The model under review builds one solid part; all positions refer to its coordinate system, in mm. Face numbers are marked on the shaded views. A direction names the side the tool comes from. Round coordinates to 2 decimals unless told otherwise and drop trailing zeros. Write each loop counter-clockwise with the first axis right and the second up, starting at its lowest first coordinate (ties: lowest second). Pieces come first, ordered by that corner, then holes. Notation, with made-up numbers: (54, -31.75) - (70, -31.75) arc R33 cw to (70, 1.25) - close; hole circle Ø2 at (28, 42). An arc over 180 degrees is marked (long way). Return JSON: item names as keys, results as strings.
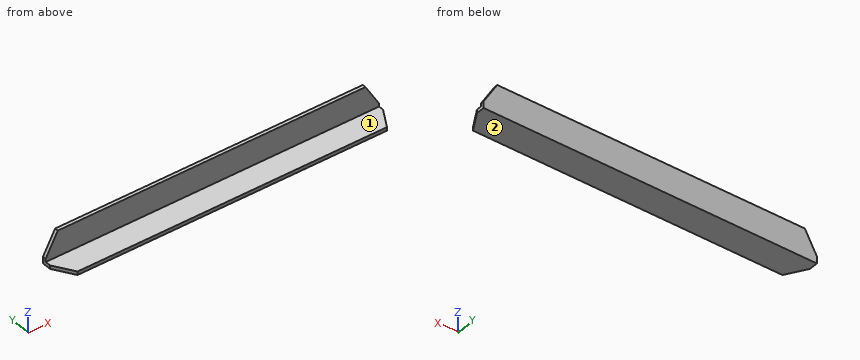
from build123d import *

# Parameters (mm, degrees)
F0_W      = 294.42918
F0_H      = 25.4
F1_DEPTH  = 3.048
F2_W      = 294.42918
F2_H      = 3.048
F3_DEPTH  = 22.352
F5_DEPTH  = 25.4
F7_DEPTH  = 25.4
F9_DEPTH  = 25.4
F11_DEPTH = 25.4


with BuildPart() as f1:
    # F0 (on Front) → F1 (new body)
    with BuildSketch(Plane.XZ):
        with Locations((147.21459, 12.7)):
            Rectangle(F0_W, F0_H)
    extrude(amount=F1_DEPTH)

    # F2 (on face) → F3 (join)
    with BuildSketch(Plane.XZ.offset(3.048)):
        with Locations((147.21459, 1.524)):
            Rectangle(F2_W, F2_H)
    extrude(amount=F3_DEPTH)

    # F4 (on face) → F5 (cut)
    with BuildSketch(Plane.XZ.offset(3.048)):
        Polygon((0, 5.934239), (10.683293, 25.4), (4.401662, 35.47851), (-15.100691, 25.4), align=None)
    extrude(amount=-F5_DEPTH, mode=Mode.SUBTRACT)

    # F6 (on face) → F7 (cut)
    with BuildSketch(Plane.XY.offset(3.048)):
        Polygon((13.454681, -30.058125), (0, -8.04578), (-4.952007, -25.4), (9.960025, -44.26622), align=None)
    extrude(amount=-F7_DEPTH, mode=Mode.SUBTRACT)

    # F8 (on face) → F9 (cut)
    with BuildSketch(Plane.XY.offset(3.048)):
        Polygon((299.843073, 0), (294.42918, -7.468464), (280.858219, -30.611685), (297.753662, -36.44076), align=None)
    extrude(amount=-F9_DEPTH, mode=Mode.SUBTRACT)

    # F10 (on face) → F11 (cut)
    with BuildSketch(Plane.XZ.offset(3.048)):
        Polygon((279.356599, 30.402403), (294.42918, 5.696148), (301.659763, 3.048), (311.673284, 34.467302), align=None)
    extrude(amount=-F11_DEPTH, mode=Mode.SUBTRACT)


solid = f1.part
(1) Add section C-C (z = 14.5). Write out the cut boundary in (x, y), plus the area to 3 significant figures.
Filled in:
{"outline": "(4.7, -3.05) - (289.06, -3.05) - (289.06, 0) - (4.7, 0) - close", "area": "867 mm2"}
(2) For the marked faces 1 and 2, list the 3-axis set-ups (+Z, -Z, +X, -X, +Y, -Y) from which the entire face can be reached by the end or side of a thin tool; tool diameter is ignored.
Filled in:
{"face 1": "+Z, +X, -X, -Y", "face 2": "-Z, +X, -X, +Y, -Y"}
(3) Clearance check with flat-ended pins moving along their axes: pin 1 Ø12 at (x, z) = (218, 22) entering from -Y; pin 2 Ø8 at (y, z) = (-16, 8) entering from +X; pin 3 Ø1 at (x, y) = (33, -17.5) entering from +Z. State where each tip first meets the part, or that it passes through.
Filled in:
{"pin 1": "stops at y = -3.05", "pin 2": "passes through", "pin 3": "stops at z = 3.05"}
(4) Wall thickness on line 1 (Z direction, x = 136, y = -3.25); line 2 (Y direction, x = 204.5, z = 6.75); line 3 (X direction, y = -16.25, z = 2.5): over which ranges is each line inside the solid? List them lowest first.
Filled in:
{"line 1": "z = 0 to 3.05", "line 2": "y = -3.05 to 0", "line 3": "x = 5.01 to 289.28"}
(5) Add section B-B (y = -20). Write out the cut boundary in (x, z).
Filled in:
{"outline": "(7.31, 0) - (287.08, 0) - (287.08, 3.05) - (7.31, 3.05) - close"}
(6) Add section A-A (x = 204). Write out the cut boundary in (y, z).
Filled in:
{"outline": "(-25.4, 0) - (0, 0) - (0, 25.4) - (-3.05, 25.4) - (-3.05, 3.05) - (-25.4, 3.05) - close"}
